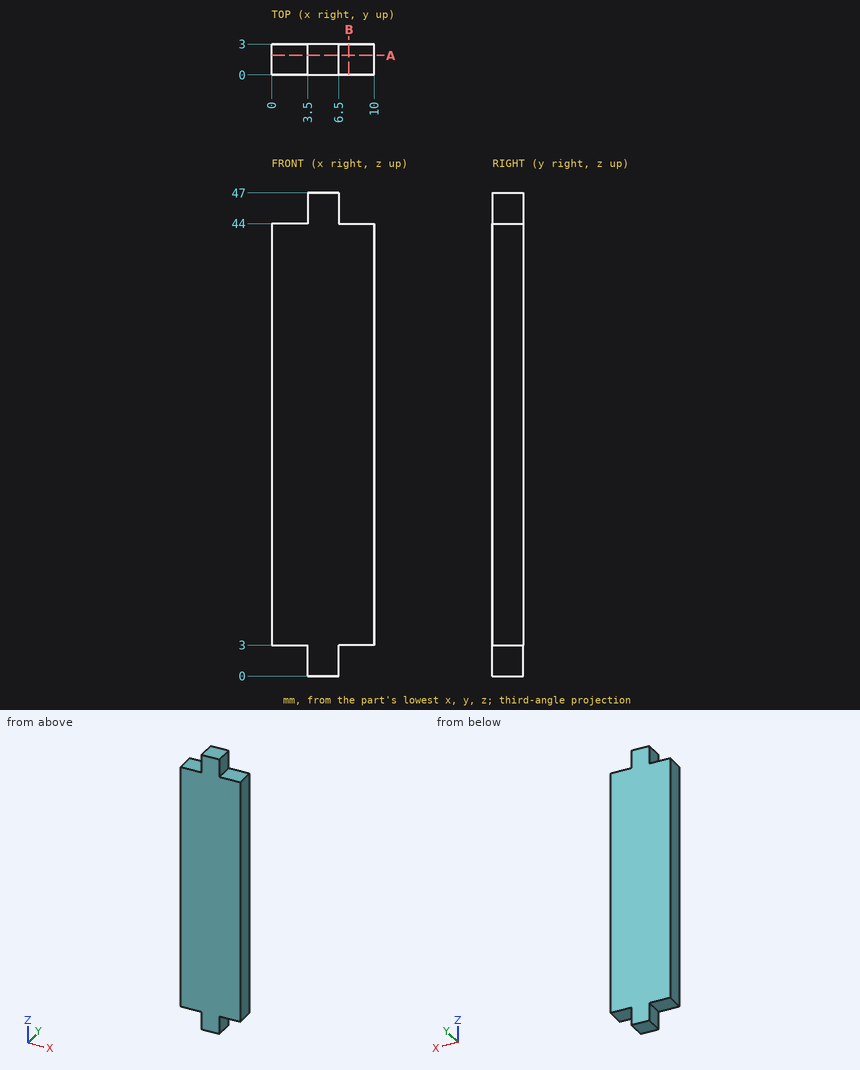
The figure shows three views and two pictorial views of one solid part (mm, origin at its lowest corner). Answer the questions. Give positions to 0.01 mm unless a question says otherwise; leave off trailing zeros. Order: outer loops, then holes, each group sorted by start corner. A loop starts at its lowest first (then second) coordinate and runs counter-clockwise, first axis right, second up. Notation, with made-up numbers: (-1.75, 51.25) -> (45.25, 51.25) arc R28 ccw to (45.25, 78.25) -> close; hole circle Ø9 at (30, -14.5). An arc over 180 degrees is marked (long way). Answer as CSV lines item,"result". Start each with the question number.
(1) Section A-A, the plane y = 1.9 is taken. Write down the section's boundary in (x, z).
(2) Consider line 1 along Z through (x, y) = (6.75, 1.7). Determine where the line is inside the solid, lowest interval first.
(3) Section B-B, the plane x = 7.5 is taken. Write down the section's boundary in (y, z).
(4) Each of these flat-tipped pins is pushed along its axis until it touches: pin 1 Ø1.5 at (x, z) = (1.5, 29.5) entering from -Y; pin 2 Ø1.5 at (y, z) = (1.5, 45.5) entering from +X; pin 3 Ø1.5 at (y, z) = (2, 2) entering from -X. Where does it stop, or does it pass through?
Entries:
1,outline,"(0, 3) -> (3.5, 3) -> (3.5, 0) -> (6.5, 0) -> (6.5, 3) -> (10, 3) -> (10, 44) -> (6.5, 44) -> (6.5, 47) -> (3.5, 47) -> (3.5, 44) -> (0, 44) -> close"
2,line 1,"3 to 44"
3,outline,"(0, 3) -> (3, 3) -> (3, 44) -> (0, 44) -> close"
4,pin 1,"y = 0"
4,pin 2,"x = 6.5"
4,pin 3,"x = 3.5"
